Design review of the part shown in the three views and the two pictorial views. Dimensions are in mm from the part's minimum x, y and z. Coordinates: 2 decimals unless noted, no trailing zeros. Write each loop counter-clockwise with the first axis right and the second up, starting at its lowest first coordinate (ties: lowest second). Pieces come first, ordered by that corner, then holes. Notation, with made-up numbers: (69.25, 11) - (121.25, 11) arc R35 cw to (121.25, 49) - close; hole circle Ø3 at (-23.75, 57). An arc over 180 degrees is marked (long way). Return JSON: item names as keys, results as strings. Group by question number.
(1) To check wall thickness, follow L1, parallel to Y at x = 12.5, z = 3.7; L2, parallel to X at y = 16.5, z = 5.15; L3, parallel to X at y = 20.75, z = 5.1. State the ranges of each line that lie inside material, in increasing order. Write a range as from..to.
(2) We need section B-B on y = 12.5. State the section outline as (x, z) points, then the cut area to 3 significant figures.
(3) We need section C-C on z = 5.65. State the section outline as (x, y) points.
(4) For pin 1 Ø3 at (x, y) = (12.5, 4) entering from -Z, flat-tipped, find the tip position at first contact; note if it passes through.
(5) Draft analysis for pull direction Y (two halves, no side actions). For the marked faces 1, 2 and 3, state which applies: released by +Y, released by -Y, zero draft, split by the parting line, or undercut.
(6) We need section A-A on x = 12.5. State the section outline as (y, z) points, then the cut area to 3 significant figures.
(7) We need section D-D on x = 17. State the section outline as (y, z) points.
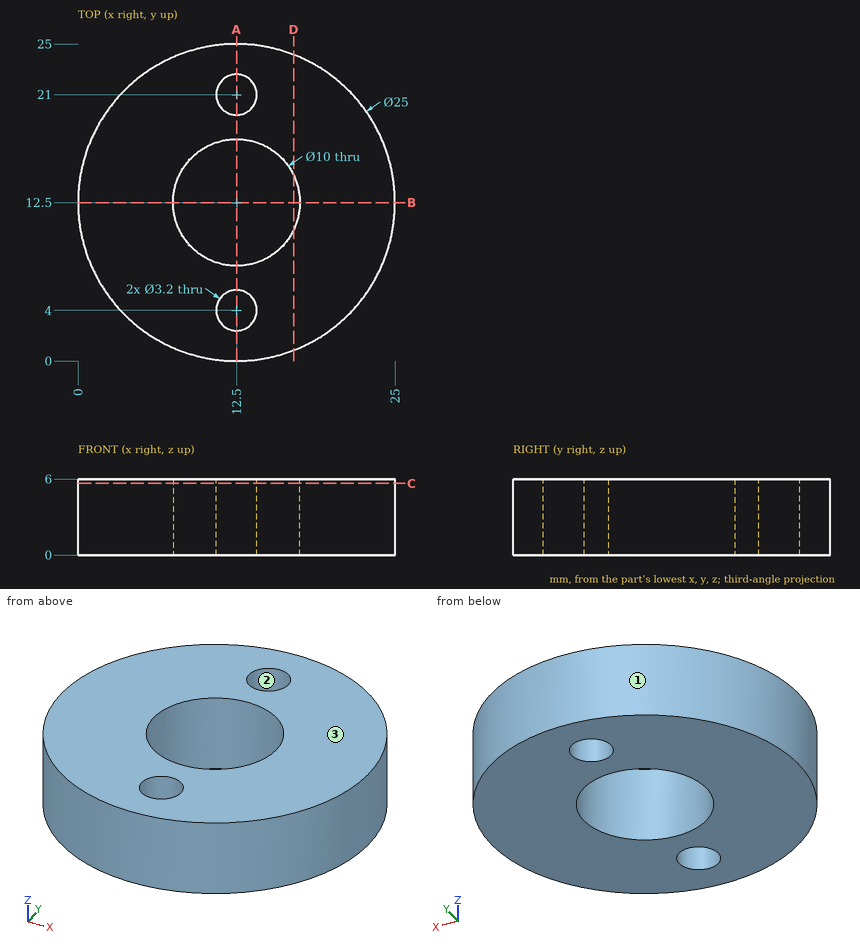
Ans:
{
 "1": {"L1": "0..2.4, 5.6..7.5, 17.5..19.4, 22.6..25", "L2": "0.66..9.5, 15.5..24.34", "L3": "3.11..10.92, 14.08..21.89"},
 "2": {"outline": "(0, 0) - (7.5, 0) - (7.5, 6) - (0, 6) - close; (17.5, 0) - (25, 0) - (25, 6) - (17.5, 6) - close", "area": "90.0 mm²"},
 "3": {"outline": "circle Ø25 at (12.5, 12.5); hole circle Ø10 at (12.5, 12.5); hole circle Ø3.2 at (12.5, 4); hole circle Ø3.2 at (12.5, 21)"},
 "4": {"pin 1": "through"},
 "5": {"face 1": "split by the parting line", "face 2": "undercut", "face 3": "zero draft"},
 "6": {"outline": "(0, 0) - (2.4, 0) - (2.4, 6) - (0, 6) - close; (5.6, 0) - (7.5, 0) - (7.5, 6) - (5.6, 6) - close; (17.5, 0) - (19.4, 0) - (19.4, 6) - (17.5, 6) - close; (22.6, 0) - (25, 0) - (25, 6) - (22.6, 6) - close", "area": "51.6 mm²"},
 "7": {"outline": "(0.84, 0) - (10.32, 0) - (10.32, 6) - (0.84, 6) - close; (14.68, 0) - (24.16, 0) - (24.16, 6) - (14.68, 6) - close"}
}
